Input: part model. Units: mm. Frame: model coordinates. A direction names the side the tool comes from. Give positions to 0.01 mm unless a question says otherwise; leave off trailing zeros. Loops run counter-clockwise (first coordinate to the right, second up) from the corner with the lowest first, then second, coordinate; pieces in that order, holes last. Notation, with made-up numbers: M 19.5,18 L 25.5,18 A14 cw 25.5,23 Z; hole C 11,-26 d2. An arc over 180 degrees is marked long. Use a Markdown table: item, result. Add a question column.
from build123d import *

# Parameters (mm, degrees)
SKETCH2_R           = 40
BOSS_EXTRUDE1_DEPTH = 4
SKETCH3_W           = 2
SKETCH3_H           = 1


with BuildPart() as part:
    # Sketch2 → Boss-Extrude1 (new body)
    with BuildSketch(Plane(origin=(0, 0, 0), x_dir=(0, 0, -1), z_dir=(1, 0, 0))):
        Circle(SKETCH2_R)
        with BuildLine():
            Line((-2, 1.5), (2, 1.5))
            ThreePointArc((2, 1.5), (2.5, 0), (2, -1.5))
            Line((2, -1.5), (-2, -1.5))
            ThreePointArc((-2, -1.5), (-2.5, 0), (-2, 1.5))
        make_face(mode=Mode.SUBTRACT)
        with BuildLine():
            ThreePointArc((-15.90290373, 31.178480607), (-30.419515024, 17.310491203), (-34.927407255, -2.253047362))
            ThreePointArc((-34.927407255, -2.253047362), (-20.583361548, -1.767102241), (-6.968299733, 2.77358952))
            ThreePointArc((-6.968299733, 2.77358952), (-4.209992791, 6.206928443), (0, 7.5))
            ThreePointArc((0, 7.5), (-6.227172355, 20.497298183), (-15.90290373, 31.178480607))
        make_face(mode=Mode.SUBTRACT)
        with BuildLine():
            ThreePointArc((5.886148851, 4.64792983), (8.761325342, 18.709265117), (15.512507376, 31.374545653))
            ThreePointArc((15.512507376, 31.374545653), (30.201082646, 17.68882718), (34.952808122, -1.81692168))
            ThreePointArc((34.952808122, -1.81692168), (21.122165812, -3.688321149), (7.313076649, -1.664004186))
            ThreePointArc((7.313076649, -1.664004186), (7.315395834, 1.653778642), (5.886148851, 4.64792983))
        make_face(mode=Mode.SUBTRACT)
        with BuildLine():
            ThreePointArc((1.082150882, -7.42151935), (11.822036206, -16.942162875), (19.414899879, -29.12149829))
            ThreePointArc((19.414899879, -29.12149829), (0.218432378, -34.999318383), (-19.049904392, -29.361558927))
            ThreePointArc((-19.049904392, -29.361558927), (-13.755262718, -16.448171602), (-5.097608221, -5.501308065))
            ThreePointArc((-5.097608221, -5.501308065), (-2.2254836, -7.162207952), (1.082150882, -7.42151935))
        make_face(mode=Mode.SUBTRACT)
    extrude(amount=BOSS_EXTRUDE1_DEPTH)

    # Sketch3 → Cut-Revolve1 (revolve, cut)
    with BuildSketch(Plane.XY):
        with Locations((2, 39.5)):
            Rectangle(SKETCH3_W, SKETCH3_H)
    revolve(axis=Axis((-1.599073018, 0, 0), (1, 0, 0)), mode=Mode.SUBTRACT)

    # Sketch4 → Revolve1 (revolve)
    with BuildSketch(Plane.XY):
        Polygon((3, 40), (2, 39), (3, 39), align=None)
    revolve(axis=Axis((0, 0, 0), (1, 0, 0)))


solid = part.part
1) Pull-direction query (X, two-part tool) for faces 1 (the cylindrical face through (2, -16.8, -11.7)), 2 (the cylindrical face through (1.507, -5.077, 38.668)), 3 (the flat face through (0, -8, -8)); classes: pulls with the +X half, pulls with the -X half, needs draft (parallel to the pull), parting line crosses it, or undercut.
2) Section query B-B, the plane z = -12. State how many separate pieces and enclosed holes the cut face has, and give its area (3 significant figures).
3) Contact query for flat-ended pins moving along their axis: P1, Ø1, axis at x = 2, z = -21.5, coming from the -Y side; P2, Ø1, axis at x = 2, z = 14, coming from the +Y side; P3, Ø1, axis at x = 3, z = 9, coming from the +Y side; P4, Ø2, axis at y = -19, z = 20.5, coming from the -X side. Output: stop coordinate, or through.
4) Reachability of faces 4 (the flat face through (1, -38.3, -8.7)), 5 (the cylindrical face through (1.97, -7.15, 2.27)) from +Z, -Z, +X, -X, +Y, -Y: full face, straight path, thin tool, end or side. Return the list, or none.
5) Ray query, line 1 (Y direction, x = 1.25, z = -0.5); line 2 (Z direction, x = 0.5, y = 12); line 3 (Y direction, x = 3.1, z = -1.5). Return the intervals inside material, ascending. Write a range as [from, to].
6) Section query A-A, the plane y = 0. Return the cut outline in (x, z).
Entries:
| question | item | result |
|---|---|---|
| 1 | face 1 | needs draft |
| 1 | face 2 | undercut |
| 1 | face 3 | pulls with the -X half |
| 2 | separate pieces | 3 |
| 2 | enclosed holes | 0 |
| 2 | area | 125 mm² |
| 3 | P1 | stops at y = -33.22 |
| 3 | P2 | stops at y = 36.97 |
| 3 | P3 | stops at y = 39.09 |
| 3 | P4 | stops at x = 0 |
| 4 | face 4 | none |
| 4 | face 5 | +X, -X |
| 5 | line 1 | y = [-39, -35], [-7.48, -1.5], [1.5, 39] |
| 5 | line 2 | z = [-38.16, -32.88], [-6.86, 1.64], [32.88, 38.16] |
| 5 | line 3 | y = [-39.97, -34.97], [-7.7, -1.5], [1.5, 39.97] |
| 6 | outline | M 0,-40 L 1,-40 L 1,-39 L 2,-39 L 3,-40 L 4,-40 L 4,-35 L 0,-35 Z; M 0,-7.5 L 4,-7.5 L 4,-2.5 L 0,-2.5 Z; M 0,2.5 L 4,2.5 L 4,13.65 L 0,13.65 Z; M 0,35 L 4,35 L 4,40 L 3,40 L 2,39 L 1,39 L 1,40 L 0,40 Z |
